The listing builds one solid part. Answer for the finished solid, in the listing's coordinates (mm). A direction names the side the tool comes from. Give positions to 0.01 mm unless a question says otherwise; leave off trailing zeros. Order: outer loops, then holes, each group sorted by start corner. A loop starts at its lowest first (then second) coordinate and runs counter-clockwise, first axis right, second up. Notation, with made-up numbers: (55, -30.75) - (90, -30.75) arc R27 ccw to (90, 1.25) - close; hole circle Ø7 at (28.5, -36.5). An arc over 180 degrees is marked (long way). Answer in a Markdown table with one row per item. Add a question column.
```python
from build123d import *

# Parameters (mm, degrees)
CROQUIS2_W              = 115.37
CROQUIS2_H              = 45.3
CROQUIS2_R              = 3.25
CROQUIS2_R_2            = 1.65
SALIENTE_EXTRUIR1_DEPTH = 21.4
CROQUIS6_W              = 48.38
CROQUIS6_H              = 35.8
CORTAR_EXTRUIR1_DEPTH   = 18.4
CROQUIS9_W              = 9.3
CROQUIS9_H              = 15
CROQUIS9_R              = 1.65
SALIENTE_EXTRUIR4_DEPTH = 3
REDONDEO8_R             = 4.65
CROQUIS7_W              = 115.37
CROQUIS7_H              = 3.9
SALIENTE_EXTRUIR3_DEPTH = 5
REDONDEO2_R             = 5
CORTAR_EXTRUIR2_DEPTH   = 133.828035068
REDONDEO9_R             = 2
CROQUIS12_W             = 57.67
CROQUIS12_H             = 20.44
CORTAR_EXTRUIR3_DEPTH   = 18.4
REDONDEO10_R            = 1


with BuildPart() as part:
    # Croquis2 → Saliente-Extruir1 (new body)
    with BuildSketch(Plane(origin=(0, 0, 0), x_dir=(1, 0, 0), z_dir=(0, 1, 0))):
        with Locations((57.685, 22.65)):
            Rectangle(CROQUIS2_W, CROQUIS2_H)
        with Locations(Location((57.685, 19.5, 0), (0, 0, 270))):
            Circle(CROQUIS2_R, mode=Mode.SUBTRACT)
        with Locations(Location((75.685, 19.5, 0), (0, 0, 270))):
            Circle(CROQUIS2_R_2, mode=Mode.SUBTRACT)
        with Locations(Location((39.685, 19.5, 0), (0, 0, 90))):
            Circle(CROQUIS2_R_2, mode=Mode.SUBTRACT)
    extrude(amount=SALIENTE_EXTRUIR1_DEPTH)

    # Croquis6 → Cortar-Extruir1 (cut)
    with BuildSketch(Plane(origin=(0, 21.4, 0), x_dir=(1, 0, 0), z_dir=(0, 1, 0))):
        with Locations((57.685, 27.4)):
            Rectangle(CROQUIS6_W, CROQUIS6_H)
    extrude(amount=-CORTAR_EXTRUIR1_DEPTH, mode=Mode.SUBTRACT)

    # Croquis9 → Saliente-Extruir4 (add)
    # profile 1 of 4: a face of its own
    with BuildSketch(Plane(origin=(0, 21.4, 0), x_dir=(1, 0, 0), z_dir=(0, 1, 0))):
        with Locations((86.52, 52.8)):
            Rectangle(CROQUIS9_W, CROQUIS9_H)
        with Locations(Location((86.52, 55.65, 0), (0, 0, 270))):
            Circle(CROQUIS9_R, mode=Mode.SUBTRACT)
    # profile 2 of 4: a face of its own
    with BuildSketch(Plane(origin=(0, 21.4, 0), x_dir=(1, 0, 0), z_dir=(0, 1, 0))):
        with Locations((28.85, 52.8)):
            Rectangle(CROQUIS9_W, CROQUIS9_H)
        with Locations(Location((28.85, 55.65, 0), (0, 0, 90))):
            Circle(CROQUIS9_R, mode=Mode.SUBTRACT)
    # profile 3 of 4: a face of its own
    with BuildSketch(Plane(origin=(0, 21.4, 0), x_dir=(1, 0, 0), z_dir=(0, 1, 0))):
        with Locations((69.345, -7.5)):
            Rectangle(CROQUIS9_W, CROQUIS9_H)
        with Locations(Location((69.345, -10.35, 0), (0, 0, 270))):
            Circle(CROQUIS9_R, mode=Mode.SUBTRACT)
    # profile 4 of 4: a face of its own
    with BuildSketch(Plane(origin=(0, 21.4, 0), x_dir=(1, 0, 0), z_dir=(0, 1, 0))):
        with Locations((46.025, -7.5)):
            Rectangle(CROQUIS9_W, CROQUIS9_H)
        with Locations(Location((46.025, -10.35, 0), (0, 0, 90))):
            Circle(CROQUIS9_R, mode=Mode.SUBTRACT)
    extrude(amount=-SALIENTE_EXTRUIR4_DEPTH)

    # Redondeo8
    redondeo8_edges = [part.edges().sort_by_distance(p)[0] for p in [
        (73.995, 19.9, 15),
        (64.695, 19.9, 15),
        (41.375, 19.9, 15),
        (50.675, 19.9, 15),
        (91.17, 19.9, -60.3),
        (81.87, 19.9, -60.3),
        (33.5, 19.9, -60.3),
        (24.2, 19.9, -60.3),
    ]]
    fillet(redondeo8_edges, radius=REDONDEO8_R - 0.0001)  # a hair under: the kernel refuses the full size

    # Croquis7 → Saliente-Extruir3 (add)
    with BuildSketch(Plane.XZ):
        with Locations((57.685, -43.35)):
            Rectangle(CROQUIS7_W, CROQUIS7_H)
        with Locations((57.685, -1.95)):
            Rectangle(CROQUIS7_W, CROQUIS7_H)
    extrude(amount=SALIENTE_EXTRUIR3_DEPTH)

    # Redondeo2
    redondeo2_edges = [part.edges().sort_by_distance(p)[0] for p in [
        (0, 8.2, 0),
        (0, 8.2, -45.3),
        (115.37, 8.2, -45.3),
        (115.37, 8.2, 0),
    ]]
    fillet(redondeo2_edges, radius=REDONDEO2_R)

    # Croquis11 → Cortar-Extruir2 (cut, through all)
    with BuildSketch(Plane(origin=(0, 21.4, 0), x_dir=(1, 0, 0), z_dir=(0, 1, 0))):
        with BuildLine():
            Line((115.37, 18.647739407), (115.37, 5))
            ThreePointArc((115.37, 5), (113.905533906, 1.464466094), (110.37, 0))
            Line((110.37, 0), (97.550134045, 0))
            ThreePointArc((97.550134045, 0), (105.831202258, 9.924815779), (115.37, 18.647739407))
        make_face()
        with BuildLine():
            Line((0, 18.647739407), (0, 5))
            ThreePointArc((0, 5), (1.464466094, 1.464466094), (5, 0))
            Line((5, 0), (17.819865955, 0))
            ThreePointArc((17.819865955, 0), (9.538797742, 9.924815779), (0, 18.647739407))
        make_face()
    extrude(amount=-CORTAR_EXTRUIR2_DEPTH, mode=Mode.SUBTRACT)

    # Redondeo9
    redondeo9_edges = [part.edges().sort_by_distance(p)[0] for p in [
        (97.550134045, 8.2, 0),
        (115.37, 10.7, -18.647739407),
        (0, 10.7, -18.647739407),
        (17.819865955, 8.2, 0),
    ]]
    fillet(redondeo9_edges, radius=REDONDEO9_R)

    # Croquis12 → Cortar-Extruir3 (cut)
    with BuildSketch(Plane(origin=(0, 21.4, 0), x_dir=(1, 0, 0), z_dir=(0, 1, 0))):
        with Locations((57.685, 19.72)):
            Rectangle(CROQUIS12_W, CROQUIS12_H)
    extrude(amount=-CORTAR_EXTRUIR3_DEPTH, mode=Mode.SUBTRACT)

    # Redondeo10
    redondeo10_edges = [part.edges().sort_by_distance(p)[0] for p in [
        (33.495, 12.2, -29.94),
        (81.875, 12.2, -29.94),
    ]]
    fillet(redondeo10_edges, radius=REDONDEO10_R)


solid = part.part
```
(1) Each of these flat-tipped pins is pushed along its axis until it touches: P1, Ø2, axis at x = 37, y = 5, coming from the -Z side; P2, Ø3, axis at x = 39.685, z = -19.5, coming from the +Y side; P3, Ø5.5, axis at y = 12.5, z = -16.5, coming from the -X side; P4, Ø1.5, axis at y = 20, z = -50, coming from the +X side. Where does it stop, or does it pass through?
(2) The mould has two halves that part along Z. Classify faces 1 (the face through (40.7, 1.5, -18.2)), 2 (the face through (0, 11, -30)), 3 (the face through (1.43, 8.02, -43.8)): +Z half, -Z half, draft (parallel to the pull), parting line (faces both ways), or undercut.
(3) Find section C-C, the plane x = 66. Write down the section's boundary in (y, z), plus the area to 3 significant figures.
(4) Find section D-D, the plane x = 104. Write down the section's boundary in (y, z).
(5) For faces 4 (the face through (57, 12, -9.5)), 5 (the face through (66.02, 19.88, 13.6)), 6 (the face through (57, 0, -23)), determine the directions among +Z, -Z, +X, -X, +Y, -Y from which every point of the face is accessible in a straight line to the end or side of a thin tool.
(6) Find section A-A, the plane z = -47.5. Write down the section's boundary in (x, y), plus the area to 3 significant figures.
(7) Straight lines are drawn through the part: line 1 (X direction, y = 19.4, z = 10.35) (3 decimals); line 2 (X direction, y = 19.1, z = -55.65); line 3 (Z direction, x = 63.5, y = -1.75). For each, find the intervals that lie inside material, in ascending order.
Answer key:
| question | item | result |
|---|---|---|
| 1 | P1 | z = -9.5 |
| 1 | P2 | through |
| 1 | P3 | x = 0.03 |
| 1 | P4 | x = 91.17 |
| 2 | face 1 | undercut |
| 2 | face 2 | draft |
| 2 | face 3 | -Z half |
| 3 | outline | (-5, -45.3) - (3, -45.3) - (3, -9.5) - (21.4, -9.5) - (21.4, 13.58) - (18.4, 13.58) - (18.4, 0) - (-5, 0) - (-5, -3.9) - (0, -3.9) - (0, -41.4) - (-5, -41.4) - close |
| 3 | area | 390 mm² |
| 4 | outline | (-5, -45.3) - (21.4, -45.3) - (21.4, -7.95) - (0, -7.95) - (0, -41.4) - (-5, -41.4) - close |
| 5 | face 4 | +Y |
| 5 | face 5 | +Z, +Y, -Y |
| 5 | face 6 | +X, -X, -Y |
| 6 | outline | (24.2, 18.4) - (33.5, 18.4) - (33.5, 21.4) - (24.2, 21.4) - close; (81.87, 18.4) - (91.17, 18.4) - (91.17, 21.4) - (81.87, 21.4) - close |
| 6 | area | 55.8 mm² |
| 7 | line 1 | 41.375 to 44.375, 47.675 to 50.675, 64.695 to 67.695, 70.995 to 73.995 |
| 7 | line 2 | 24.2 to 27.2, 30.5 to 33.5, 81.87 to 84.87, 88.17 to 91.17 |
| 7 | line 3 | -45.3 to -41.4, -3.9 to 0 |
